```python
from build123d import *

# Parameters (mm, degrees)
SKETCH1_R           = 1.75
BOSS_EXTRUDE1_DEPTH = 1


with BuildPart() as part:
    # Sketch1 → Boss-Extrude1 (new body)
    with BuildSketch(Plane(origin=(0, 0, 0), x_dir=(1, 0, 0), z_dir=(0, 1, 0))):
        with BuildLine():
            Line((132.75, -5.75), (2.75, -5.75))
            ThreePointArc((2.75, -5.75), (-4.321067812, -2.821067812), (-7.25, 4.25))
            Line((-7.25, 4.25), (-7.25, 39.25))
            ThreePointArc((-7.25, 39.25), (-4.321067812, 46.321067812), (2.75, 49.25))
            Line((2.75, 49.25), (132.75, 49.25))
            ThreePointArc((132.75, 49.25), (139.821067812, 46.321067812), (142.75, 39.25))
            Line((142.75, 39.25), (142.75, 4.25))
            ThreePointArc((142.75, 4.25), (139.821067812, -2.821067812), (132.75, -5.75))
        make_face()
        with Locations(Location((0, 0, 0), (0, 0, 270))):
            Circle(SKETCH1_R, mode=Mode.SUBTRACT)
        with Locations(Location((0, 43.5, 0), (0, 0, 270))):
            Circle(SKETCH1_R, mode=Mode.SUBTRACT)
        with Locations(Location((135.5, 43.5, 0), (0, 0, 270))):
            Circle(SKETCH1_R, mode=Mode.SUBTRACT)
        with Locations(Location((135.5, 0, 0), (0, 0, 270))):
            Circle(SKETCH1_R, mode=Mode.SUBTRACT)
        with BuildLine():
            Line((130.25, 40.016443463), (130.25, 44.666666667))
            Line((130.25, 44.666666667), (5.25, 44.666666667))
            Line((5.25, 44.666666667), (5.25, 40.020251196))
            ThreePointArc((5.25, 40.020251196), (0.205636176, 37.930807287), (-1.883807733, 32.886443463))
            Line((-1.883807733, 32.886443463), (-1.883807733, 10.613556537))
            ThreePointArc((-1.883807733, 10.613556537), (0.205636176, 5.569192713), (5.25, 3.479748804))
            Line((5.25, 3.479748804), (5.25, -1.166666667))
            Line((5.25, -1.166666667), (130.25, -1.166666667))
            Line((130.25, -1.166666667), (130.25, 3.483556537))
            ThreePointArc((130.25, 3.483556537), (135.29167135, 5.571885187), (137.38, 10.613556537))
            Line((137.38, 10.613556537), (137.38, 32.886443463))
            ThreePointArc((137.38, 32.886443463), (135.29167135, 37.928114813), (130.25, 40.016443463))
        make_face(mode=Mode.SUBTRACT)
    extrude(amount=BOSS_EXTRUDE1_DEPTH)


solid = part.part
```
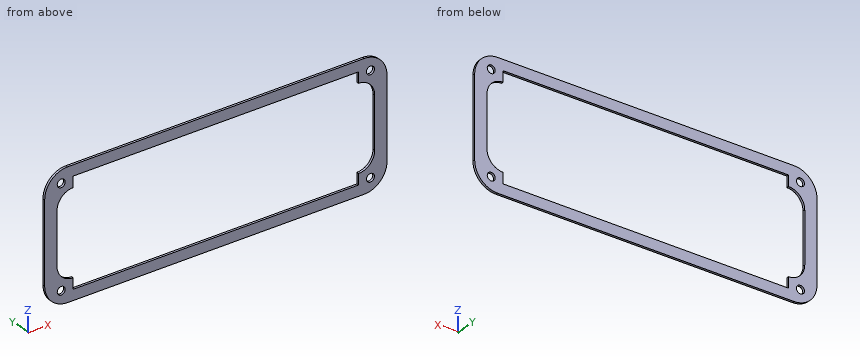
Read the model definition and answer for the solid it produces. Units are mm, in the model's axes. Give positions to 0.01 mm unless a question says otherwise; leave off trailing zeros. Write each loop counter-clockwise with the first axis right and the second up, starting at its lowest first coordinate (ties: lowest second). Pieces come first, ordered by that corner, then holes. Notation, with made-up numbers: (-38.5, -10.5) -> (-3.5, -10.5) arc R23 cw to (-3.5, 4.5) -> close; hole circle Ø9 at (9, 19). An arc over 180 degrees is marked (long way). Answer as a JSON object with one key per item and string values.
1) Section A-A on z = -27 is taken. Write down the section's boundary in (x, y), then the cut area to 3 significant figures.
Findings below:
{"outline": "(-7.25, 0) -> (-1.88, 0) -> (-1.88, 1) -> (-7.25, 1) -> close; (137.38, 0) -> (142.75, 0) -> (142.75, 1) -> (137.38, 1) -> close", "area": "10.7 mm^2"}
2) Straight lines are drawn through the part: probe 1 along X at (y, z) = (0.8, -19.5); probe 2 along X at (y, z) = (0.3, 1); probe 3 along X at (y, z) = (0.45, 0). For each, find the intervals that lie inside material, in ascending order. Write a range as from..to.
Findings below:
{"probe 1": "x = -7.25..-1.88, 137.38..142.75", "probe 2": "x = -5.76..-1.44, 1.44..5.25, 130.25..134.06, 136.94..141.26", "probe 3": "x = -6.3..-1.75, 1.75..5.25, 130.25..133.75, 137.25..141.8"}
3) Section C-C on x = 104 is taken. Write down the section's boundary in (y, z).
Findings below:
{"outline": "(0, -49.25) -> (1, -49.25) -> (1, -44.67) -> (0, -44.67) -> close; (0, 1.17) -> (1, 1.17) -> (1, 5.75) -> (0, 5.75) -> close"}
4) Section B-B on y = 0.3 is taken. Write down the section's boundary in (x, z).
Findings below:
{"outline": "(-7.25, -39.25) arc R10 ccw to (2.75, -49.25) -> (132.75, -49.25) arc R10 ccw to (142.75, -39.25) -> (142.75, -4.25) arc R10 ccw to (132.75, 5.75) -> (2.75, 5.75) arc R10 ccw to (-7.25, -4.25) -> close; hole (-1.88, -32.89) arc R7.13 ccw to (5.25, -40.02) -> (5.25, -44.67) -> (130.25, -44.67) -> (130.25, -40.02) arc R7.13 ccw to (137.38, -32.89) -> (137.38, -10.61) arc R7.13 ccw to (130.25, -3.48) -> (130.25, 1.17) -> (5.25, 1.17) -> (5.25, -3.48) arc R7.13 ccw to (-1.88, -10.61) -> close; hole circle Ø3.5 at (0, -43.5); hole circle Ø3.5 at (0, 0); hole circle Ø3.5 at (135.5, -43.5); hole circle Ø3.5 at (135.5, 0)"}
5) Section D-D on x = 135.5 is taken. Write down the section's boundary in (y, z), then the cut area to 3 significant figures.
Findings below:
{"outline": "(0, -48.86) -> (1, -48.86) -> (1, -45.25) -> (0, -45.25) -> close; (0, -41.75) -> (1, -41.75) -> (1, -37.71) -> (0, -37.71) -> close; (0, -5.79) -> (1, -5.79) -> (1, -1.75) -> (0, -1.75) -> close; (0, 1.75) -> (1, 1.75) -> (1, 5.36) -> (0, 5.36) -> close", "area": "15.3 mm^2"}
